```python
from build123d import *

# Parameters (mm, degrees)
F0_R     = 20.32
F1_DEPTH = 25.4


with BuildPart() as f1:
    # F0 (on Front) → F1 (new body)
    with BuildSketch(Plane.XZ):
        with BuildLine():
            ThreePointArc((3.191482456, -25.1986991675), (19.05549336, -16.794289887), (25.4, 0))
            ThreePointArc((25.4, 0), (19.05549336, 16.794289887), (3.191482456, 25.1986991675))
            ThreePointArc((3.191482456, 25.1986991675), (-25.4, 0), (3.191482456, -25.1986991675))
        make_face()
        Circle(F0_R, mode=Mode.SUBTRACT)
        with BuildLine():
            ThreePointArc((3.191482456, 25.1986991675), (19.05549336, 16.794289887), (25.4, 0))
            ThreePointArc((25.4, 0), (19.05549336, -16.794289887), (3.191482456, -25.1986991675))
            Line((3.191482456, -25.1986991675), (77.238430457, -15.8204557155))
            ThreePointArc((77.238430457, -15.8204557155), (68.4813106902, 0), (77.238430457, 15.8204557155))
            Line((77.238430457, 15.8204557155), (3.191482456, 25.1986991675))
        make_face()
        with BuildLine():
            ThreePointArc((105.8193823808, 0), (96.1915572628, 16.333689356), (77.238430457, 15.8204557155))
            Line((77.238430457, 15.8204557155), (88.965929824, 14.3351366427))
            ThreePointArc((88.965929824, 14.3351366427), (97.9907117184, 9.5540027185), (101.6, 0))
            ThreePointArc((101.6, 0), (97.9907117184, -9.5540027185), (88.965929824, -14.3351366427))
            Line((88.965929824, -14.3351366427), (77.238430457, -15.8204557155))
            ThreePointArc((77.238430457, -15.8204557155), (96.1915572628, -16.333689356), (105.8193823808, 0))
        make_face()
        with BuildLine():
            Line((88.965929824, 14.3351366427), (77.238430457, 15.8204557155))
            ThreePointArc((77.238430457, 15.8204557155), (68.4813106902, 0), (77.238430457, -15.8204557155))
            Line((77.238430457, -15.8204557155), (88.965929824, -14.3351366427))
            ThreePointArc((88.965929824, -14.3351366427), (72.7006930711, 0), (88.965929824, 14.3351366427))
        make_face()
    extrude(amount=F1_DEPTH)


solid = f1.part
```
For this review, take the finished solid that the model builds, in its own axes (mm). A direction names the side the tool comes from. Round coordinates to 2 decimals unless told otherwise and drop trailing zeros. Order: outer loops, then holes, each group sorted by start corner. A loop starts at its lowest first (then second) coordinate and runs counter-clockwise, first axis right, second up. Notation, with made-up numbers: (-23, -19) -> (27, -19) arc R21 cw to (27, 20) -> close; hole circle Ø7 at (24, 12). An arc over 180 degrees is marked (long way). Use a Markdown table: item, result.
Item 1: For line 1 along X through (y, z) = (-7.5, -12); line 2 along Z through (x, y) = (0, -19.5); line 3 along X through (y, z) = (-21, 10), list the stretches that pass through material, from the lowest coordinate up. Write a range as [from, to].
Resolved:
| item | result |
|---|---|
| line 1 | x = [-22.39, -16.4], [16.4, 79.1], [95.2, 101.45] |
| line 2 | z = [-25.4, -20.32], [20.32, 25.4] |
| line 3 | x = [-23.35, -17.69], [17.69, 76.72], [97.58, 102.92] |
Item 2: For pin 1 (8 mm diameter, centred on x = 19.5, y = -12.5, fed in from -Z); pin 2 (1.5 mm diameter, centred on y = -10.5, z = -11.5, fed in from +X); pin 3 (4 mm diameter, centred on x = 13, y = -16.5, fed in from -Z), all flat-tipped, find the tip position at first contact; note any pin that passes through.
Resolved:
| item | result |
|---|---|
| pin 1 | stops at z = -23.64 |
| pin 2 | stops at x = 102.41 |
| pin 3 | stops at z = -24.21 |
Item 3: Draft analysis for pull direction X (two halves, no side actions). For faces 3 (the flat face through (39, -25.4, 0)), 4 (the flat face through (40.733, -12.522, 20.444)), state which applies: +X half, -X half, draft (parallel to the pull), parting line (faces both ways), or undercut.
Resolved:
| item | result |
|---|---|
| face 3 | draft |
| face 4 | undercut |
Item 4: Machinability: for faces 1 (the cylindrical face through (-2.645, -12.522, 20.147)), 2 (the flat face through (39.697, -12.522, -20.575)), which of the approach directions +Z, -Z, +X, -X, +Y, -Y give a long, thin tool a straight path to every point of the face, cutting with its end or side? Answer none if there is none.
Resolved:
| item | result |
|---|---|
| face 1 | +Y, -Y |
| face 2 | -Z, +Y, -Y |
Item 5: Take a section at D-D (x = 58). State the section outline as (y, z) points, plus the area to 3 significant figures.
Resolved:
| item | result |
|---|---|
| outline | (-25.4, -18.26) -> (0, -18.26) -> (0, 18.26) -> (-25.4, 18.26) -> close |
| area | 927 mm² |
Item 6: Take a section at B-B (x = 0). State the section outline as (y, z) points, plus the area to 3 significant figures.
Resolved:
| item | result |
|---|---|
| outline | (-25.4, -25.4) -> (0, -25.4) -> (0, -20.32) -> (-25.4, -20.32) -> close; (-25.4, 20.32) -> (0, 20.32) -> (0, 25.4) -> (-25.4, 25.4) -> close |
| area | 258 mm² |
Item 7: Take a section at C-C (z = -11). State the section outline as (x, y) points.
Resolved:
| item | result |
|---|---|
| outline | (-22.89, -25.4) -> (-17.09, -25.4) -> (-17.09, 0) -> (-22.89, 0) -> close; (17.09, -25.4) -> (77.78, -25.4) -> (77.78, 0) -> (17.09, 0) -> close; (96.52, -25.4) -> (102.23, -25.4) -> (102.23, 0) -> (96.52, 0) -> close |
Item 8: Take a section at A-A (y = -21). State the section outline as (x, z) points, plus the area to 3 significant figures.
Resolved:
| item | result |
|---|---|
| outline | (3.19, -25.2) -> (77.24, -15.82) arc R18.67 ccw (long way) to (77.24, 15.82) -> (3.19, 25.2) arc R25.4 ccw (long way) to start; hole circle Ø40.64 at (0, 0); hole circle Ø28.9 at (87.15, 0) |
| area | 3,160 mm² |
